The drawing under review shows one solid part. Ordinate dimensions are in mm from its lowest x, y, z. A direction names the side the tool comes from. Round coordinates to 2 decimals unless told otherwise and drop trailing zeros. Order: outer loops, then holes, each group sorted by start corner. A loop starts at its lowest first (then second) coordinate and runs counter-clockwise, first axis right, second up.
1) Consider section B-B (x = 14.5). Give the boundary of the cut face in (y, z), then the cut area to 3 significant figures.
2) Consider section D-D (x = 1.5). Give the boundary of the cut face in (y, z).
3) Consider section A-A (z = 26.5). Give the boundary of the cut face in (x, y).
4) Machinability: for the marked faces 1 and 2, which of the approach directions +Z, -Z, +X, -X, +Y, -Y give a long, thin tool a straight path to every point of the face, cutting with its end or side? Answer none if there is none.
5) To check wall thickness, follow L1, parallel to Z at x = 14.75, y = 15.25; L2, parallel to X at y = 4.5, z = 25.5; L3, parallel to Y at x = 4.75, z = 19. State the ranges of each line that lie inside material, in increasing order.
6) Consider section C-C (y = 18.25). Give the boundary of the cut face in (x, z).
7) Clearance check with flat-ended pins moving along their axes: P1, Ø4, axis at x = 14.5, z = 13.5, coming from the -Y side (1 decimal); P2, Ø6, axis at y = 12.5, z = 13.5, coming from the -X side (3 decimals); P3, Ø1, axis at x = 3, y = 15.5, coming from the -Z side. State where each tip first meets the part, or that it passes through.
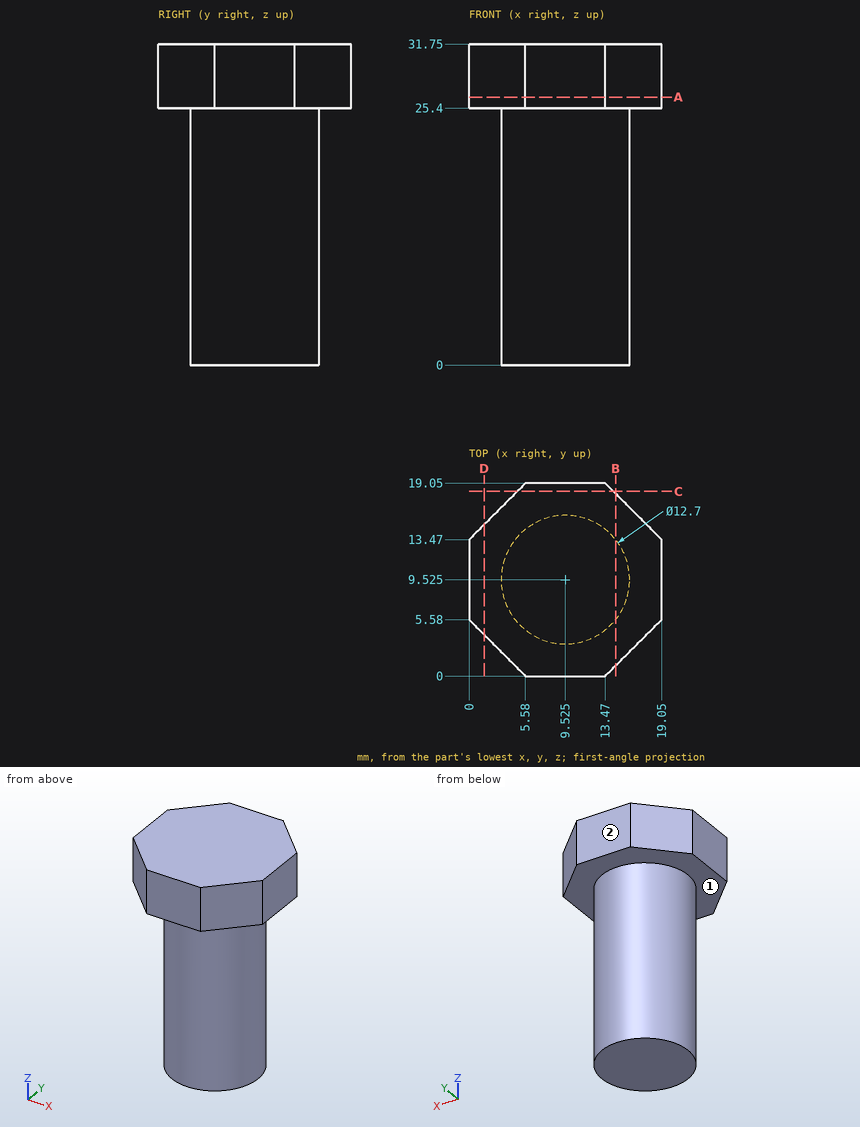
Answer below:
1. outline: (1.03, 25.4) - (5.58, 25.4) - (5.58, 0) - (13.47, 0) - (13.47, 25.4) - (18.02, 25.4) - (18.02, 31.75) - (1.03, 31.75) - close
1. area: 308 mm2
2. outline: (4.08, 25.4) - (14.97, 25.4) - (14.97, 31.75) - (4.08, 31.75) - close
3. outline: (0, 5.58) - (5.58, 0) - (13.47, 0) - (19.05, 5.58) - (19.05, 13.47) - (13.47, 19.05) - (5.58, 19.05) - (0, 13.47) - close
4. face 1: -Z
4. face 2: +Z, -Z, +X, -X, +Y
5. L1: z = 25.4 to 31.75
5. L2: x = 1.08 to 17.97
5. L3: y = 5.34 to 13.71
6. outline: (4.78, 25.4) - (14.27, 25.4) - (14.27, 31.75) - (4.78, 31.75) - close
7. P1: stops at y = 3.9
7. P2: stops at x = 3.175
7. P3: stops at z = 25.4
